The listing builds one solid part. Answer for the finished solid, in the listing's coordinates (mm). Face numbers are marked on the shaded views. A direction names the side the tool comes from. Round coordinates to 2 decimals unless told otherwise and drop trailing zeros. Loops run counter-clockwise (first coordinate to the right, second up) from the corner with the lowest first, then second, coordinate; pieces in that order, holes last. Notation, with made-up numbers: (70.25, -40) -> (127.25, -40) arc R11 cw to (127.25, -19) -> close; hole circle Ø10 at (30, 15.5). An arc over 180 degrees is marked (long way). Answer in a Markdown table with one row per item. Add a question column.
```python
from build123d import *

# Parameters (mm, degrees)
SKETCH1_W               = 6
SKETCH1_H               = 6
BOSS_EXTRUDE1_DEPTH     = 9
SKETCH2_R               = 1.5
BOSS_EXTRUDE2_DEPTH     = 3
CUT_EXTRUDE1_DEPTH      = 13.727922061
CUT_EXTRUDE1_DEPTH_BACK = 13.727922061
SKETCH3_R               = 0.68
BOSS_EXTRUDE3_START     = 38
SKETCH3_3_R             = 0.92
SKETCH3_3_R_2           = 0.68
BOSS_EXTRUDE3_DEPTH     = 38
SKETCH4_R               = 2
CUT_EXTRUDE2_DEPTH      = 8
CUT_EXTRUDE3_START      = -1
SKETCH6_W               = 6
SKETCH6_H               = 6
SKETCH6_R               = 2.8
CUT_EXTRUDE3_DEPTH      = 3


with BuildPart() as part:
    # Sketch1 → Boss-Extrude1 (new body)
    with BuildSketch(Plane(origin=(0, 0, 0), x_dir=(1, 0, 0), z_dir=(0, 1, 0))):
        Rectangle(SKETCH1_W, SKETCH1_H)
    extrude(amount=BOSS_EXTRUDE1_DEPTH)

    # Sketch2 → Boss-Extrude2 (add)
    with BuildSketch(Plane(origin=(0, 9, 0), x_dir=(1, 0, 0), z_dir=(0, 1, 0))):
        with Locations(Location((0, 0, 0), (0, 0, 270))):
            Circle(SKETCH2_R)
    extrude(amount=BOSS_EXTRUDE2_DEPTH)

    # Sketch3 → Cut-Extrude1 (cut, two sides: drawn at the far end of the back side and taken through both)
    with BuildSketch(Plane(origin=(0, 12, 0), x_dir=(1, 0, 0), z_dir=(0, 1, 0)).offset(-CUT_EXTRUDE1_DEPTH_BACK)):
        with Locations(Location((0, 0, 0), (0, 0, 270))):
            Circle(SKETCH3_R)
    extrude(amount=CUT_EXTRUDE1_DEPTH + CUT_EXTRUDE1_DEPTH_BACK, mode=Mode.SUBTRACT)

    # Sketch3<3> → Boss-Extrude3 (add)
    with BuildSketch(Plane(origin=(0, 12, 0), x_dir=(1, 0, 0), z_dir=(0, 1, 0)).offset(BOSS_EXTRUDE3_START)):
        with Locations(Location((0, 0, 0), (0, 0, 270))):
            Circle(SKETCH3_3_R)
        with Locations(Location((0, 0, 0), (0, 0, 270))):
            Circle(SKETCH3_3_R_2, mode=Mode.SUBTRACT)
    extrude(amount=-BOSS_EXTRUDE3_DEPTH)

    # Sketch4 → Cut-Extrude2 (cut)
    with BuildSketch(Plane.XZ):
        with Locations(Location((0, 0, 0), (0, 0, 270))):
            Circle(SKETCH4_R)
    extrude(amount=-CUT_EXTRUDE2_DEPTH, mode=Mode.SUBTRACT)

    # Sketch6 → Cut-Extrude3 (cut)
    with BuildSketch(Plane.XZ.offset(CUT_EXTRUDE3_START)):
        Rectangle(SKETCH6_W, SKETCH6_H)
        with Locations(Location((0, 0, 0), (0, 0, 270))):
            Circle(SKETCH6_R, mode=Mode.SUBTRACT)
    extrude(amount=-CUT_EXTRUDE3_DEPTH, mode=Mode.SUBTRACT)


solid = part.part
```
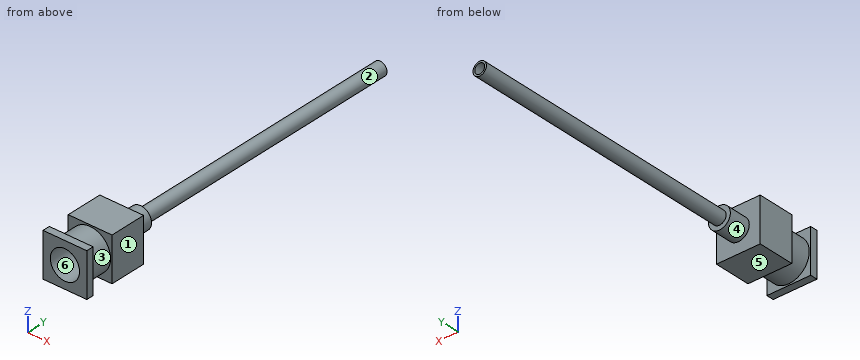
Item 1: Consider L1, parallel to Y at x = -2.7, z = -1.5; L2, parallel to X at y = 5, z = 0; L3, parallel to X at y = 11, z = 0. Determine where each line is inside the solid, lowest interval first. Write a range as from..to.
Item 2: Section A-A, the plane x = 0 is taken. Write down the section's boundary in (y, z).
Item 3: For the marked faces 1, 2 and 3, determine the directions among +Z, -Z, +X, -X, +Y, -Y from which every point of the face is accessible in a straight line to the end or side of a thin tool.
Item 4: Flat-ended cylindrical pins translate along their axes: P1, Ø2, axis at y = 11, z = 0, coming from the +X side; P2, Ø3, axis at x = 0.5, z = 0.5, coming from the -Y side; P3, Ø1.5, axis at y = 30.5, z = 1, coming from the -X side; P4, Ø3, axis at x = -0.5, y = 23, coming from the -Z side. Find the tip coordinate at first contact, or state that the pin passes through.
Item 5: Section C-C, the plane y = 36 is taken. Write down the section's boundary in (x, z), and give its area (3 significant figures).
Item 6: Section B-B, the plane z = 0 is taken. Write down the section's boundary in (x, y).
Item 7: The mould has two halves that part along Z. Classify the marked faces 4, 5 and 6: +Z half, -Z half, draft (parallel to the pull), parting line (faces both ways), or undercut.
Here are the results:
| question | item | result |
|---|---|---|
| 1 | L1 | y = 0..1, 4..9 |
| 1 | L2 | x = -3..-2, 2..3 |
| 1 | L3 | x = -1.5..-0.68, 0.68..1.5 |
| 2 | outline | (0, -3) -> (1, -3) -> (1, -2.8) -> (4, -2.8) -> (4, -3) -> (9, -3) -> (9, -1.5) -> (12, -1.5) -> (12, -0.92) -> (50, -0.92) -> (50, -0.68) -> (8, -0.68) -> (8, -2) -> (0, -2) -> close; (0, 2) -> (8, 2) -> (8, 0.68) -> (50, 0.68) -> (50, 0.92) -> (12, 0.92) -> (12, 1.5) -> (9, 1.5) -> (9, 3) -> (4, 3) -> (4, 2.8) -> (1, 2.8) -> (1, 3) -> (0, 3) -> close |
| 3 | face 1 | +Z, -Z, +X, +Y, -Y |
| 3 | face 2 | +Y |
| 3 | face 3 | none |
| 4 | P1 | stops at x = 1.5 |
| 4 | P2 | stops at y = 0 |
| 4 | P3 | stops at x = -0.89 |
| 4 | P4 | stops at z = -0.92 |
| 5 | outline | circle Ø1.84 at (0, 0); hole circle Ø1.36 at (0, 0) |
| 5 | area | 1.21 mm² |
| 6 | outline | (-3, 0) -> (-2, 0) -> (-2, 8) -> (-0.68, 8) -> (-0.68, 50) -> (-0.92, 50) -> (-0.92, 12) -> (-1.5, 12) -> (-1.5, 9) -> (-3, 9) -> (-3, 4) -> (-2.8, 4) -> (-2.8, 1) -> (-3, 1) -> close; (0.68, 8) -> (2, 8) -> (2, 0) -> (3, 0) -> (3, 1) -> (2.8, 1) -> (2.8, 4) -> (3, 4) -> (3, 9) -> (1.5, 9) -> (1.5, 12) -> (0.92, 12) -> (0.92, 50) -> (0.68, 50) -> close |
| 7 | face 4 | parting line |
| 7 | face 5 | -Z half |
| 7 | face 6 | undercut |
